Input: part model. Units: mm. Frame: model coordinates. A direction names the side the tool comes from. Give positions to 0.01 mm unless a question says otherwise; leave off trailing zeros. Loops run counter-clockwise (first coordinate to the right, second up) from the corner with the lowest first, then second, coordinate; pieces in that order, holes last.
from build123d import *

# Parameters (mm, degrees)
SKETCH_1_R      = 4.75
EXTRUDE_1_DEPTH = 1.3
SKETCH_2_R      = 2.5
EXTRUDE_2_DEPTH = 10
CHAMFER_1_SIZE  = 0.5
FILLET_1_SIZE   = 1
FILLET_1_SIZE_2 = 2


with BuildPart() as part:
    # 草图1 → 凸台-拉伸1 (new body)
    with BuildSketch(Plane(origin=(0, 0, 0), x_dir=(1, 0, 0), z_dir=(0, 1, 0))):
        with Locations(Location((0, 0, 0), (0, 0, 270))):
            Circle(SKETCH_1_R)
        Polygon((0, -1.732050808), (1.5, -0.866025404), (1.5, 0.866025404), (0, 1.732050808), (-1.5, 0.866025404), (-1.5, -0.866025404), align=None, mode=Mode.SUBTRACT)
    extrude(amount=EXTRUDE_1_DEPTH)

    # 草图2 → 凸台-拉伸2 (add)
    with BuildSketch(Plane(origin=(0, 1.3, 0), x_dir=(1, 0, 0), z_dir=(0, 1, 0))):
        with Locations(Location((0, 0, 0), (0, 0, 270))):
            Circle(SKETCH_2_R)
    extrude(amount=EXTRUDE_2_DEPTH)

    # 倒角1
    chamfer_1_edges = [part.edges().sort_by_distance(p)[0] for p in [
        (0, 11.3, -2.5),
    ]]
    chamfer(chamfer_1_edges, length=CHAMFER_1_SIZE)

    # 圆角1
    # an asymmetric fillet: 2, 1 mm, written as the material it takes off along each edge
    with BuildSketch(Plane(origin=(0, 0, 0), x_dir=(0, 0, 1), z_dir=(-1, 0, 0))) as fillet_1_piece_1:
        with BuildLine():
            Bezier((4.75, FILLET_1_SIZE), (4.75, 0), (4.75 - FILLET_1_SIZE_2, 0), weights=[1, 0.707106781, 1])
            Line((4.75 - FILLET_1_SIZE_2, 0), (4.75, 0))
            Line((4.75, 0), (4.75, FILLET_1_SIZE))
        make_face()
    revolve(axis=Axis((0, 0, 0), (0, 1, 0)), mode=Mode.SUBTRACT)


solid = part.part
(1) Mould query, pull axis X, two halves, no side actions, for faces 1 (the flat face through (0, 11.3, 0)), 2 (the flat face through (0, 1.3, 0)), 3 (the cylindrical face through (-2.44, 5.98, -0.54)). Classes: +X half, -X half, draft (parallel to the pull), parting line (faces both ways), or undercut.
Values follow:
face 1: draft
face 2: undercut
face 3: parting line
(2) Pin query (flat end, axial travel): pin 1 Ø2 at (x, y) = (-1.5, 6) entering from +Z; pin 2 Ø1 at (y, z) = (8, 0.5) entering from -X. Return the tip coordinate at first contact, or that it passes through.
Values follow:
pin 1: stops at z = 2.45
pin 2: stops at x = -2.5
(3) Ray query, probe 1 along Y at (x, z) = (-0.75, -1.25); probe 2 along Z at (x, y) = (1.5, 8); probe 3 along Y at (x, z) = (1.25, -2.5). Return the intervals inside material, ascending.
Values follow:
probe 1: y = 1.3 to 11.3
probe 2: z = -2 to 2
probe 3: y = 0 to 1.3
(4) Cut plane A-A (y = 10.25). Return the cut outline in (x, z), and give its area (3 significant figures).
Values follow:
outline: circle Ø5 at (0, 0)
area: 19.6 mm2
(5) Reachability of faces 4 (the flat face through (0, 0, 2)), 5 (the flat face through (-2, 1.3, 2)), 6 (the flat face through (-1.5, 1, 0)) from +Z, -Z, +X, -X, +Y, -Y: full face, straight path, thin tool, end or side. Return the list, or none.
Values follow:
face 4: +Z, -Z, +X, -X, -Y
face 5: +Y
face 6: -Y
